```python
from build123d import *

# Parameters (mm, degrees)
F1_DEPTH = 3.5
F2_R     = 3.49999


# Not quite as in the source:
# - a fillet or chamfer is up to 0.001 mm smaller than in the source, because OpenCascade refuses the exact size


with BuildPart() as f1:
    # F0 (on Front) → F1 (new body, symmetric)
    with BuildSketch(Plane.XZ):
        Polygon((192, 0), (0, 0), (0, -24.9), (32.5, -24.9), (192, -2.9), align=None)
    extrude(amount=F1_DEPTH, both=True)

    # F2 (radius 3.5 in the source; OpenCascade refuses exactly that, so slightly less here)
    f2_edges = [f1.edges().sort_by_distance(p)[0] for p in [
        (96, -3.5, 0),
        (96, 3.5, 0),
        (16.25, -3.5, -24.9),
        (16.25, 3.5, -24.9),
    ]]
    fillet(f2_edges, radius=F2_R)


solid = f1.part
```
Can you work these out from the model? Positions are in its coordinate system, mm. Coordinates: 2 decimals unless noted, no trailing zeros. Write each loop counter-clockwise with the first axis right and the second up, starting at its lowest first coordinate (ties: lowest second). Pieces come first, ordered by that corner, then holes. Notation, with made-up numbers: (8.5, 80) - (50.5, 80) arc R26 ccw to (50.5, 109) - close; hole circle Ø7 at (49.25, 88). An arc over 180 degrees is marked (long way). Return JSON: item names as keys, results as strings.
Q1. If we section it at C-C (z = -7.5): Please give me the cut outline in (x, y).
Computed values:
{"outline": "(0, -3.5) - (158.65, -3.5) - (158.65, 3.5) - (0, 3.5) - close"}
Q2. Please list where these lines run through material, in increasing order: L1, parallel to Z at x = 19, y = 0.5; L2, parallel to Z at x = 182, y = -2; L3, parallel to Y at x = 184.5, z = -2.75. Write a range as from..to.
Computed values:
{"L1": "z = -24.86..-0.04", "L2": "z = -4.28..-0.63", "L3": "y = -3.42..3.42"}
Q3. I'm going to push flat-ended pins straight in: pin 1 Ø2 at (x, y) = (153, 0.5) entering from +Z; pin 2 Ø2 at (x, y) = (167.5, 0.5) entering from -Z. Where does each tip first touch, or does it pass through?
Computed values:
{"pin 1": "stops at z = 0", "pin 2": "stops at z = -6.42"}
Q4. If we section it at B-B (y = -2): Please give me the cut outline in (x, z), then the cut area to 3 significant figures.
Computed values:
{"outline": "(0, -24.27) - (37.05, -24.27) - (192, -2.9) - (192, -0.63) - (0, -0.63) - close", "area": "2,880 mm2"}
